```python
from build123d import *

# Parameters (mm, degrees)
SKETCH1_W           = 41.5
SKETCH1_H           = 20.5
SKETCH1_R           = 1.25
BOSS_EXTRUDE1_DEPTH = 40
CHAMFER1_SIZE       = 5
CHAMFER1_SIZE2      = 8
SKETCH2_W           = 7.25
SKETCH2_H           = 20.506105109
SKETCH2_R           = 2.25
BOSS_EXTRUDE2_DEPTH = 2.5
SKETCH3_W           = 50.5
SKETCH3_H           = 2
BOSS_EXTRUDE3_DEPTH = 0.8
FILLET1_R           = 1
SKETCH4_R           = 6.75
BOSS_EXTRUDE4_DEPTH = 2
CHAMFER2_SIZE2      = 1
CHAMFER2_SIZE       = 2
BOSS_EXTRUDE5_DEPTH = 1.25
BOSS_EXTRUDE5_DRAFT = 30
FILLET2_R           = 1
BOSS_EXTRUDE6_START = 6
SKETCH6_R           = 3
SKETCH6_R_2         = 1.25
BOSS_EXTRUDE6_DEPTH = 6
SKETCH7_R           = 2
SKETCH7_W           = 7
SKETCH7_H           = 4.5
BOSS_EXTRUDE7_DEPTH = 5


with BuildPart() as part:
    # Sketch1 → Boss-Extrude1 (new body)
    with BuildSketch(Plane(origin=(0, 0, 0), x_dir=(1, 0, 0), z_dir=(0, 1, 0))):
        with Locations((10.75, 0)):
            Rectangle(SKETCH1_W, SKETCH1_H)
        with Locations(Location((0, 0, 0), (0, 0, 270))):
            Circle(SKETCH1_R, mode=Mode.SUBTRACT)
    extrude(amount=-BOSS_EXTRUDE1_DEPTH)

    # Chamfer1
    chamfer1_edges = [part.edges().sort_by_distance(p)[0] for p in [
        (31.5, 0, 0),
    ]]
    chamfer1_side = [part.faces().sort_by_distance(p)[0] for p in [
        (31.5, -20, 0),
    ]]
    chamfer(chamfer1_edges, length=CHAMFER1_SIZE, length2=CHAMFER1_SIZE2, reference=chamfer1_side[0])

    # Sketch2 → Boss-Extrude2 (add)
    # profile 1 of 2: a face of its own
    with BuildSketch(Plane(origin=(0, -8, 0), x_dir=(1, 0, 0), z_dir=(0, 1, 0))):
        with Locations((-13.625, -0.003052554)):
            Rectangle(SKETCH2_W, SKETCH2_H)
        with Locations(Location((-14.25, 4.996947445, 0), (0, 0, 270))):
            Circle(SKETCH2_R, mode=Mode.SUBTRACT)
        with Locations(Location((-14.25, -5.003052555, 0), (0, 0, 90))):
            Circle(SKETCH2_R, mode=Mode.SUBTRACT)
    # profile 2 of 2: a face of its own
    with BuildSketch(Plane(origin=(0, -8, 0), x_dir=(1, 0, 0), z_dir=(0, 1, 0))):
        with Locations((35.125, -0.003052554)):
            Rectangle(SKETCH2_W, SKETCH2_H)
        with Locations(Location((35.75, 4.996947445, 0), (0, 0, 90))):
            Circle(SKETCH2_R, mode=Mode.SUBTRACT)
        with Locations(Location((35.75, -5.003052555, 0), (0, 0, 270))):
            Circle(SKETCH2_R, mode=Mode.SUBTRACT)
    extrude(amount=-BOSS_EXTRUDE2_DEPTH)

    # Sketch3 → Boss-Extrude3 (add)
    with BuildSketch(Plane(origin=(0, -8, 0), x_dir=(1, 0, 0), z_dir=(0, 1, 0))):
        with Locations((10.75, 0)):
            Rectangle(SKETCH3_W, SKETCH3_H)
    extrude(amount=BOSS_EXTRUDE3_DEPTH)

    # Fillet1
    fillet1_edges = [part.edges().sort_by_distance(p)[0] for p in [
        (36, -7.6, 1),
        (36, -7.6, -1),
        (-14.5, -7.6, -1),
        (-14.5, -7.6, 1),
    ]]
    fillet(fillet1_edges, radius=FILLET1_R - 0.0001)  # a hair under: the kernel refuses the full size

    # Sketch4 → Boss-Extrude4 (add)
    with BuildSketch(Plane(origin=(0, 0, 0), x_dir=(1, 0, 0), z_dir=(0, 1, 0))):
        with Locations(Location((0, 0, 0), (0, 0, 270))):
            Circle(SKETCH4_R)
    extrude(amount=BOSS_EXTRUDE4_DEPTH)

    # Chamfer2
    chamfer2_edges = [part.edges().sort_by_distance(p)[0] for p in [
        (0, 2, -6.75),
    ]]
    chamfer2_side = [part.faces().sort_by_distance(p)[0] for p in [
        (0, 1.98, -6.75),
    ]]
    chamfer(chamfer2_edges, length=CHAMFER2_SIZE - 0.0001, length2=CHAMFER2_SIZE2 - 0.0001, reference=chamfer2_side[0])  # a hair under: the kernel refuses the full size


with BuildPart() as boss_extrude5_tool:
    # Sketch5 → Boss-Extrude5 (with draft: the straight prism first)
    with BuildSketch(Plane(origin=(0, 0, 0), x_dir=(1, 0, 0), z_dir=(0, 1, 0))):
        with BuildLine():
            ThreePointArc((13.436698586, 1.75), (11, 3), (8.563301414, 1.75))
            Line((8.563301414, 1.75), (2.982880946, 1.75))
            Line((2.982880946, 1.75), (2.982880946, -1.75))
            Line((2.982880946, -1.75), (8.563301414, -1.75))
            ThreePointArc((8.563301414, -1.75), (11, -3), (13.436698586, -1.75))
            Line((13.436698586, -1.75), (22, -1.75))
            Line((22, -1.75), (22, 1.75))
            Line((22, 1.75), (13.436698586, 1.75))
        make_face()
    extrude(amount=BOSS_EXTRUDE5_DEPTH)
    # Boss-Extrude5: the draft: its side faces are tilted about the plane it starts from
    boss_extrude5_sides = [boss_extrude5_tool.faces().sort_by_distance(p)[0] for p in [
        (11, 0.625, -3),
        (5.77309118, 0.625, -1.75),
        (2.982880946, 0.625, 0),
        (5.77309118, 0.625, 1.75),
        (11, 0.625, 3),
        (17.718349293, 0.625, 1.75),
        (22, 0.625, 0),
        (17.718349293, 0.625, -1.75),
    ]]
    draft(boss_extrude5_sides, Plane(origin=(0, 0, 0), x_dir=(1, 0, 0), z_dir=(0, 1, 0)), BOSS_EXTRUDE5_DRAFT)


with BuildPart() as part_1:
    add(part.part)

    # Boss-Extrude5: add boss_extrude5_tool
    add(boss_extrude5_tool.part)

    # Fillet2
    fillet2_edges = [part_1.edges().sort_by_distance(p)[0] for p in [
        (21.639156082, 0.625, 1.389156082),
        (21.639156082, 0.625, -1.389156082),
    ]]
    fillet(fillet2_edges, radius=FILLET2_R)

    # Sketch6 → Boss-Extrude6 (add)
    with BuildSketch(Plane(origin=(0, 0, 0), x_dir=(1, 0, 0), z_dir=(0, 1, 0)).offset(BOSS_EXTRUDE6_START)):
        with Locations(Location((0, 0, 0), (0, 0, 270))):
            Circle(SKETCH6_R)
        with Locations(Location((0, 0, 0), (0, 0, 270))):
            Circle(SKETCH6_R_2, mode=Mode.SUBTRACT)
    extrude(amount=-BOSS_EXTRUDE6_DEPTH)

    # Sketch7 → Boss-Extrude7 (add)
    with BuildSketch(Plane.ZY.offset(10)):
        with Locations((0, -22)):
            Circle(SKETCH7_R)
        with Locations((0, -33.25)):
            Rectangle(SKETCH7_W, SKETCH7_H)
    extrude(amount=BOSS_EXTRUDE7_DEPTH)


solid = part_1.part
```
Check sheet for the modelled part. Datum: model origin and axes. Units: mm. A direction names the side the tool comes from. Round coordinates to 2 decimals unless told otherwise and drop trailing zeros. Order: outer loops, then holes, each group sorted by start corner. A loop starts at its lowest first (then second) coordinate and runs counter-clockwise, first axis right, second up. Notation, with made-up numbers: (68, 62.25) - (111, 62.25) arc R27 ccw to (111, 85.25) - close; hole circle Ø6 at (88.5, 71). An arc over 180 degrees is marked (long way). Answer as CSV lines item,"result". Start each with the question number.
1) Section check C-C (x = 17). Record the cut outline in (y, z), then the cut area to 3 significant figures.
2) Tool access check on faces 4 (the face through (-15, -33, 0)), 5 (the face through (7.52, 0.62, -1.39)), 6 (the face through (-13.388, -9.232, 2.925)), 7 (the face through (0, -7.2, 0)), 8 (the face through (34, -7.2, 0)). Record the directions out of +Z, -Z, +X, -X, +Y, -Y that give a thin tool (end or side, any length) a straight path to the whole face; none if there is none.
3) Section check D-D (y = -13). Record the cut outline in (x, z).
4) Section check B-B (y = -22). Record the cut outline in (x, z).
5) Scan lines: probe 1 along X at (y, z) = (-9, 4); probe 2 along Y at (x, z) = (7, -0.25); probe 3 along Y at (x, z) = (23.5, 3.25). Record each from-to range of solid material in increasing order.
6) Depth check by flat-ended pin: pin 1 (3.5 mm diameter, centred on x = -15, z = -3.5, fed in from -Y); pin 2 (10 mm diameter, centred on x = 23, y = -28, fed in from +Z); pin 3 (12 mm diameter, centred on y = 1, z = -6.5, fed in from -X); pin 4 (4 mm diameter, centred on x = 0, z = 0, fed in from -Y). Enter the tip coordinate at first touch or a pass-through.
7) Draft check along Y on faces 1 (the face through (17.14, 0.62, -1.39)), 2 (the face through (-15, -22, 0)), 3 (the face through (0, 0, 0)). Enter one of: +Y half, -Y half, draft (parallel to the pull), parting line (faces both ways), or undercut.
Determined:
1,outline,"(-40, -10.25) - (0, -10.25) - (0, -1.75) - (1.25, -1.03) - (1.25, 1.03) - (0, 1.75) - (0, 10.25) - (-40, 10.25) - close"
1,area,"823 mm^2"
2,face 4,"+Z, -Z, -X, -Y"
2,face 5,"-Z, +Y"
2,face 6,"+Y"
2,face 7,"none"
2,face 8,"+Z, -Z, +X, +Y"
3,outline,"(-10, -10.25) - (31.5, -10.25) - (31.5, 10.25) - (-10, 10.25) - close; hole circle Ø2.5 at (0, 0)"
4,outline,"(-15, -2) - (-10, -2) - (-10, -10.25) - (31.5, -10.25) - (31.5, 10.25) - (-10, 10.25) - (-10, 2) - (-15, 2) - close; hole circle Ø2.5 at (0, 0)"
5,probe 1,"-17.25 to -16.26, -12.24 to 33.74, 37.76 to 38.75"
5,probe 2,"-40 to 1.25"
5,probe 3,"-40 to 0"
6,pin 1,"y = -35.5"
6,pin 2,"z = 10.25"
6,pin 3,"x = -10"
6,pin 4,"y = -40"
7,face 1,"+Y half"
7,face 2,"draft"
7,face 3,"undercut"
